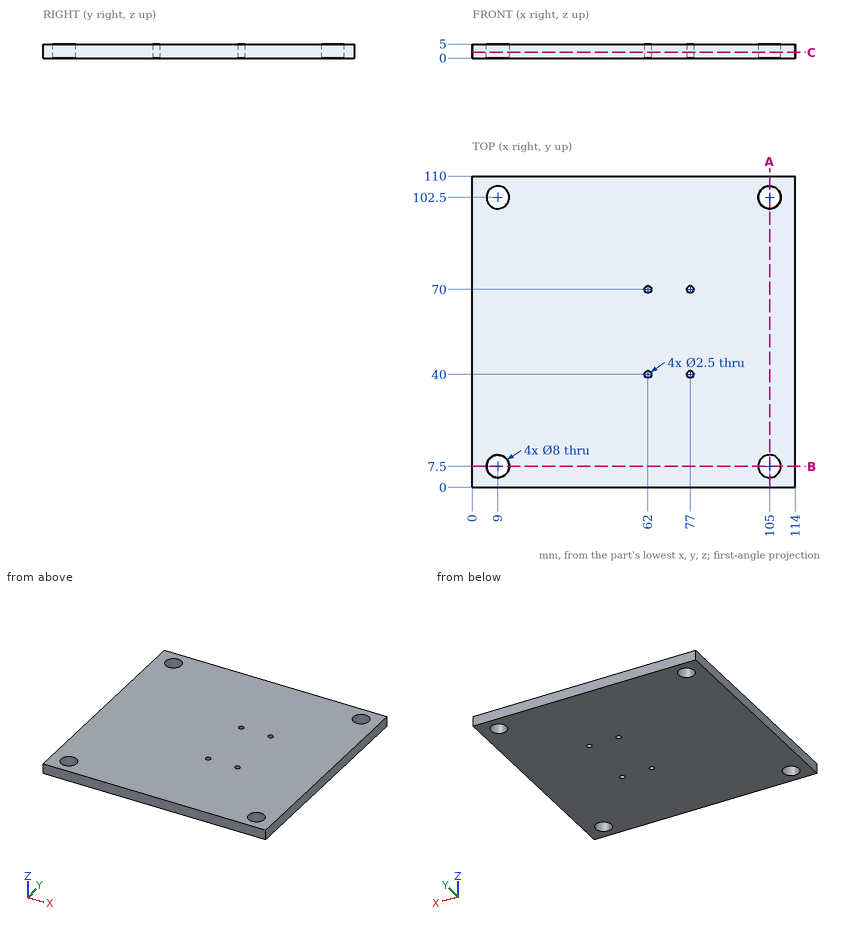
Here's the drawing with two shaded views (mm, measured from the low corner). I have some questions. Coordinates: 2 decimals unless noted, no trailing zeros. Loops run counter-clockwise (first coordinate to the right, second up) from the corner with the lowest first, then second, coordinate; pieces in that order, holes last. Notation, with made-up numbers: M 60.25,-32.5 L 71.25,-32.5 A24 ccw 71.25,-6.5 Z; hole C 24,17.5 d6. An arc over 180 degrees is marked long. Answer as CSV lines item,"result". Start each with the question number.
1. If I drill on probe 1 along Y at (x, z) = (77, 1.5); probe 2 along Y at (x, z) = (9, 2.1); probe 3 along X at (y, z) = (103, 2.9), over which ranges is the centre line in solid material (lowest first)? Write a range as [from, to].
2. Suppose I cut it at A-A, the plane x = 105. List the corners of the cut face in (y, z) for me, plus the area to 3 significant figures.
3. For pin 1 Ø2 at (x, y) = (62, 40) entering from +Z, with a flat end and sliding along its axis, tell me the tip position at first contact or that it passes through.
4. Suppose I cut it at C-C, the plane z = 2. Count the separate pieces of the cut face and the enclosed holes in it, plus the area to 3 significant figures.
5. Suppose I cut it at B-B, the plane y = 7.5. List the corners of the cut face in (x, z) for me.
Output:
1,probe 1,"y = [0, 38.75], [41.25, 68.75], [71.25, 110]"
1,probe 2,"y = [0, 3.5], [11.5, 98.5], [106.5, 110]"
1,probe 3,"x = [0, 5.03], [12.97, 101.03], [108.97, 114]"
2,outline,"M 0,0 L 3.5,0 L 3.5,5 L 0,5 Z; M 11.5,0 L 98.5,0 L 98.5,5 L 11.5,5 Z; M 106.5,0 L 110,0 L 110,5 L 106.5,5 Z"
2,area,"470 mm^2"
3,pin 1,"passes through"
4,separate pieces,"1"
4,enclosed holes,"8"
4,area,"12,300 mm^2"
5,outline,"M 0,0 L 5,0 L 5,5 L 0,5 Z; M 13,0 L 101,0 L 101,5 L 13,5 Z; M 109,0 L 114,0 L 114,5 L 109,5 Z"
